from build123d import *

# Parameters (mm, degrees)
SKETCH1_R           = 8.5
BOSS_EXTRUDE1_DEPTH = 4.4
SKETCH2_R           = 7.104307479
SKETCH2_R_2         = 6.107298405
BOSS_EXTRUDE2_DEPTH = 0.6
SKETCH3_R           = 5.8
CUT_EXTRUDE1_DEPTH  = 4
BOSS_EXTRUDE3_START = 3
SKETCH4_R           = 8.5
SKETCH4_R_2         = 7.5
BOSS_EXTRUDE3_DEPTH = 3


with BuildPart() as part:
    # Sketch1 → Boss-Extrude1 (new body)
    with BuildSketch(Plane.XY):
        Circle(SKETCH1_R)
    extrude(amount=BOSS_EXTRUDE1_DEPTH)

    # Sketch2 → Boss-Extrude2 (add)
    # profile 1 of 2: a face of its own
    with BuildSketch(Plane.XY.offset(4.4)):
        Circle(SKETCH2_R)
        Circle(SKETCH2_R_2, mode=Mode.SUBTRACT)
    # profile 2 of 2: a face of its own
    with BuildSketch(Plane.XY.offset(4.4)):
        with BuildLine():
            Line((-0.79575858, 0), (-0.79575858, 4.570978174))
            ThreePointArc((-0.79575858, 4.570978174), (0, 5.366736754), (0.79575858, 4.570978174))
            Line((0.79575858, 4.570978174), (0.79575858, 0.395496115))
            Line((0.79575858, 0.395496115), (3.622638776, -1.745931242))
            ThreePointArc((3.622638776, -1.745931242), (3.776443977, -2.860743961), (2.661631259, -3.014549161))
            Line((2.661631259, -3.014549161), (-0.480503759, -0.63430896))
            add(Edge.make_bspline(
                [(-0.79575858, 0), (-0.782929945, -0.180408247), (-0.768261528, -0.225601884), (-0.677231987, -0.437603968), (-0.573517685, -0.563848751), (-0.480503759, -0.63430896)],
                knots=[0, 0, 0, 0, 0.528419672, 0.628419672, 1, 1, 1, 1], degree=3))
        make_face()
    extrude(amount=BOSS_EXTRUDE2_DEPTH)

    # Sketch3 → Cut-Extrude1 (cut)
    with BuildSketch(Plane(origin=(0, 0, 0), x_dir=(-1, 0, 0), z_dir=(0, 0, -1))):
        Circle(SKETCH3_R)
    extrude(amount=-CUT_EXTRUDE1_DEPTH, mode=Mode.SUBTRACT)

    # Sketch4 → Boss-Extrude3 (add)
    with BuildSketch(Plane(origin=(0, 0, 0), x_dir=(-1, 0, 0), z_dir=(0, 0, -1)).offset(BOSS_EXTRUDE3_START)):
        Circle(SKETCH4_R)
        Circle(SKETCH4_R_2, mode=Mode.SUBTRACT)
    extrude(amount=-BOSS_EXTRUDE3_DEPTH)

    # Sketch6 → Cut-Revolve1 (revolve, cut)
    with BuildSketch(Plane(origin=(0, 0, 0), x_dir=(1, 0, 0), z_dir=(0, 1, 0)), mode=Mode.PRIVATE) as cut_revolve1_sk:
        Polygon((7.5, 0), (5.8, -1.7), (5.8, 0), align=None)
    revolve(cut_revolve1_sk.sketch.rotate(Axis((0, 0, -5.5), (0, 0, 1)), 180), axis=Axis((0, 0, -5.5), (0, 0, 1)), mode=Mode.SUBTRACT)


solid = part.part
The model under review builds one solid part; all positions refer to its coordinate system, in mm. A direction names the side the tool comes from. Give positions to 0.01 mm unless a question says otherwise; leave off trailing zeros. Loops run counter-clockwise (first coordinate to the right, second up) from the corner with the lowest first, then second, coordinate; pieces in that order, holes last. Notation, with made-up numbers: (-17, 22.25) -> (14, 22.25) arc R12 cw to (14, 43.25) -> close; hole circle Ø8 at (22, 30). An arc over 180 degrees is marked (long way). Answer as a JSON object with one key per item and string values. Group by question number.
Q1. Take a section at A-A (z = 2). Write out the cut boundary in (x, y).
Q2. Insertion check: pin 1 (2 mm diameter, centred on y = 5, z = 0, fed in from -X); pin 2 (6 mm diameter, centred on x = 1.5, y = 0, fed in from -Z); pin 3 (1.5 mm diameter, centred on x = 5.5, z = 1, fed in from -Y). Each pin has a flat end and moves straight along its axis. Give the tip position at first contact, or say it passes through.
Q3. Take a section at B-B (x = 0). Write out the cut boundary in (y, z).
Q4. Draft analysis for pull direction Y (two halves, no side actions). For faces 4 (the flat face through (2, 6, 5)), 5 (the flat face through (1.11, -1.84, 4.7)), 6 (the cylindrical face through (-1.54, -6.935, 4.696)), state which applies: pulls with the +Y half, pulls with the -Y half, needs draft (parallel to the pull), parting line crosses it, or undercut.
Q5. Wall thickness on line 1 along X through (y, z) = (0, 2.45); line 2 along X through (y, z) = (-2.5, 4.5); line 3 along Y through (x, z) = (0, 4.8): over which ranges is each line inside the solid? List them lowest first.
Q6. Take a section at C-C (z = -1.5). Write out the cut boundary in (x, y).
Q7. Tool access review of faces 1 (the flat face through (0, -8, -3)), 2 (the flat face through (-2, -7, 4.4)), 3 (the flat face through (0, 0, 4)): name each direction out of +Z, -Z, +X, -X, +Y, -Y from which nothing blocks a thin tool from reaching the whole face with its end or side.
Answer below:
{
 "1": {"outline": "circle Ø17 at (0, 0); hole circle Ø11.6 at (0, 0)"},
 "2": {"pin 1": "stops at x = -7.5", "pin 2": "stops at z = 4", "pin 3": "stops at y = -7.05"},
 "3": {"outline": "(-8.5, -3) -> (-7.5, -3) -> (-7.5, 0) -> (-5.8, 1.7) -> (-5.8, 4) -> (5.8, 4) -> (5.8, 1.7) -> (7.5, 0) -> (7.5, -3) -> (8.5, -3) -> (8.5, 4.4) -> (7.1, 4.4) -> (7.1, 5) -> (6.11, 5) -> (6.11, 4.4) -> (5.37, 4.4) -> (5.37, 5) -> (-1, 5) -> (-1, 4.4) -> (-6.11, 4.4) -> (-6.11, 5) -> (-7.1, 5) -> (-7.1, 4.4) -> (-8.5, 4.4) -> close"},
 "4": {"face 4": "needs draft", "face 5": "undercut", "face 6": "parting line crosses it"},
 "5": {"line 1": "x = -8.5 to -5.8, 5.8 to 8.5", "line 2": "x = -6.65 to -5.57, 1.98 to 3.93, 5.57 to 6.65", "line 3": "y = -7.1 to -6.11, -1 to 5.37, 6.11 to 7.1"},
 "6": {"outline": "circle Ø17 at (0, 0); hole circle Ø15 at (0, 0)"},
 "7": {"face 1": "-Z, +X, -X, +Y, -Y", "face 2": "+Z", "face 3": "-Z"}
}
